Could you check a few things on this model? Use its own coordinates, in mm. A direction names the side the tool comes from. Coordinates: 2 decimals unless noted, no trailing zeros. Write each loop counter-clockwise with the first axis right and the second up, starting at its lowest first coordinate (ties: lowest second). Pieces come first, ordered by that corner, then holes.
Item 1: I want a section at B-B on y = 4. Please give me the cut outline in (x, z).
Item 2: For P1, Ø8, axis at x = 29.5, z = 2, coming from the +Y side; P2, Ø4, axis at x = -2, z = -14.5, coming from the +Y side; P3, Ø1.8, axis at y = 8.5, z = 3, coming from the +X side, each with a flat end and sliding along its axis, tell me the tip position at first contact or that it passes through.
Item 3: I want a section at C-C on x = 28.5. Please give me the cut outline in (y, z).
Item 4: Thinking about a two-plate mould opening in Y: for faces 5 (the cylindrical face through (-15.62, 11.16, -3.47)), 6 (the flat face through (-14.2, 10.3, -7.7)), 7 (the flat face through (-30, 6, 0)), which applies, +Y half, -Y half, draft (parallel to the pull), parting line (faces both ways), or undercut?
Item 5: Which directions (+Z, -Z, +X, -X, +Y, -Y) give clear straight access to the entire face, cutting with the end or side of a thin tool? Please do faces 1 (the cylindrical face through (-15.62, 5.55, -3.47)), 2 (the cylindrical face through (-17.084, 9.659, -3.794)), 3 (the flat face through (25, 9, 0)), 4 (the flat face through (-25, 9, 0)).
Item 6: I want a section at A-A on z = 0. Please give me the cut outline in (x, y).
Item 7: I want a section at D-D on y = 11.25. Please give me the cut outline in (x, z), then the cut area to 3 significant figures.
Item 8: If I drill on probe 1 along X at (y, z) = (7, 0); probe 2 along X at (y, z) = (6.5, -10); probe 3 along Y at (x, z) = (10, 13), over which ranges is the centre line in solid material (lowest first)?
from build123d import *

# Parameters (mm, degrees)
SKETCH1_W           = 50
SKETCH1_H           = 50
BOSS_EXTRUDE2_DEPTH = 12
SKETCH3_R           = 16
CUT_EXTRUDE1_DEPTH  = 10
SKETCH6_R           = 10.5
CUT_EXTRUDE2_DEPTH  = 10
SKETCH9_W           = 50
SKETCH9_H           = 6
BOSS_EXTRUDE3_DEPTH = 10
SKETCH11_W          = 50
SKETCH11_H          = 6
BOSS_EXTRUDE4_DEPTH = 10
SKETCH12_R          = 2.5
CUT_EXTRUDE4_DEPTH  = 10


with BuildPart() as part:
    # Sketch1 → Boss-Extrude2 (new body)
    with BuildSketch(Plane(origin=(0, 0, 0), x_dir=(1, 0, 0), z_dir=(0, 1, 0))):
        Rectangle(SKETCH1_W, SKETCH1_H)
    extrude(amount=BOSS_EXTRUDE2_DEPTH)

    # Sketch3 → Cut-Extrude1 (cut)
    with BuildSketch(Plane(origin=(0, 12, 0), x_dir=(1, 0, 0), z_dir=(0, 1, 0))):
        with Locations(Location((0, 0, 0), (0, 0, 270))):
            Circle(SKETCH3_R)
    extrude(amount=-CUT_EXTRUDE1_DEPTH, mode=Mode.SUBTRACT)

    # Sketch5 → Cut-Revolve1 (revolve, cut)
    with BuildSketch(Plane.XY, mode=Mode.PRIVATE) as cut_revolve1_sk:
        Polygon((-16, 9), (-17.5, 9), (-17.5, 10.3), (-16, 10.3), (-15.747172999, 10.3), (-15.747172999, 9), align=None)
    revolve(cut_revolve1_sk.sketch.rotate(Axis((0, 2, 0), (0, 1, 0)), 90), axis=Axis((0, 2, 0), (0, 1, 0)), mode=Mode.SUBTRACT)

    # Sketch6 → Cut-Extrude2 (cut)
    with BuildSketch(Plane(origin=(0, 2, 0), x_dir=(1, 0, 0), z_dir=(0, 1, 0))):
        with Locations(Location((0, 0, 0), (0, 0, 270))):
            Circle(SKETCH6_R)
    extrude(amount=-CUT_EXTRUDE2_DEPTH, mode=Mode.SUBTRACT)

    # Sketch9 → Boss-Extrude3 (add)
    with BuildSketch(Plane.ZY.offset(25)):
        with Locations((0, 3)):
            Rectangle(SKETCH9_W, SKETCH9_H)
    extrude(amount=BOSS_EXTRUDE3_DEPTH)

    # Sketch11 → Boss-Extrude4 (add)
    with BuildSketch(Plane(origin=(25, 0, 0), x_dir=(0, 0, -1), z_dir=(1, 0, 0))):
        with Locations((0, 3)):
            Rectangle(SKETCH11_W, SKETCH11_H)
    extrude(amount=BOSS_EXTRUDE4_DEPTH)

    # Sketch12 → Cut-Extrude4 (cut)
    with BuildSketch(Plane(origin=(0, 6, 0), x_dir=(1, 0, 0), z_dir=(0, 1, 0))):
        with Locations(Location((-30, 15, 0), (0, 0, 270))):
            Circle(SKETCH12_R)
        with Locations(Location((-30, -15, 0), (0, 0, 90))):
            Circle(SKETCH12_R)
        with Locations(Location((30, -15, 0), (0, 0, 270))):
            Circle(SKETCH12_R)
        with Locations(Location((30, 15, 0), (0, 0, 90))):
            Circle(SKETCH12_R)
    extrude(amount=-CUT_EXTRUDE4_DEPTH, mode=Mode.SUBTRACT)


solid = part.part
Response values:
1. outline: (-35, -25) - (35, -25) - (35, 25) - (-35, 25) - close; hole circle Ø5 at (-30, -15); hole circle Ø5 at (-30, 15); hole circle Ø32 at (0, 0); hole circle Ø5 at (30, -15); hole circle Ø5 at (30, 15)
2. P1: stops at y = 6
2. P2: stops at y = 12
2. P3: stops at x = 25
3. outline: (0, -25) - (6, -25) - (6, -17) - (0, -17) - close; (0, -13) - (6, -13) - (6, 13) - (0, 13) - close; (0, 17) - (6, 17) - (6, 25) - (0, 25) - close
4. face 5: draft
4. face 6: undercut
4. face 7: +Y half
5. face 1: +Y
5. face 2: none
5. face 3: +Z, -Z, +X, +Y
5. face 4: +Z, -Z, -X, +Y
6. outline: (-35, 0) - (-10.5, 0) - (-10.5, 2) - (-16, 2) - (-16, 9) - (-17.5, 9) - (-17.5, 10.3) - (-16, 10.3) - (-16, 12) - (-25, 12) - (-25, 6) - (-35, 6) - close; (10.5, 0) - (35, 0) - (35, 6) - (25, 6) - (25, 12) - (16, 12) - (16, 10.3) - (17.5, 10.3) - (17.5, 9) - (16, 9) - (16, 2) - (10.5, 2) - close
7. outline: (-25, -25) - (25, -25) - (25, 25) - (-25, 25) - close; hole circle Ø32 at (0, 0)
7. area: 1,700 mm2
8. probe 1: x = -25 to -16, 16 to 25
8. probe 2: x = -25 to -12.49, 12.49 to 25
8. probe 3: y = 0 to 9, 10.3 to 12
